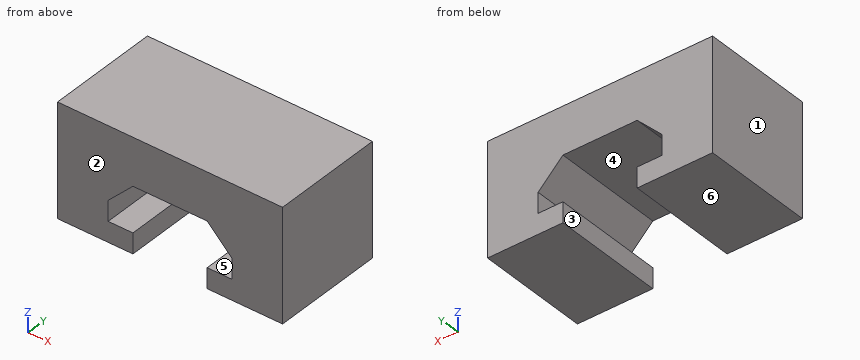
```python
from build123d import *

# Parameters (mm, degrees)
SKETCH_W     = 20
SKETCH_H     = 10
PAD_DEPTH    = 10
POCKET_DEPTH = 10.001


with BuildPart() as part:
    # Sketch → Pad (new body)
    with BuildSketch(Plane.XZ):
        with Locations((0, 5)):
            Rectangle(SKETCH_W, SKETCH_H)
    extrude(amount=PAD_DEPTH)

    # Sketch001 (on Face6 of Pad) → Pocket (cut, through all)
    with BuildSketch(Plane.XZ.offset(10)):
        Polygon((-3.3, 0), (3.3, 0), (3.3, 1.8), (5.5, 1.8), (5.5, 3.6), (3.3, 5.8), (-3.3, 5.8), (-5.5, 3.6), (-5.5, 1.8), (-3.3, 1.8), align=None)
    extrude(amount=-POCKET_DEPTH, mode=Mode.SUBTRACT)


solid = part.part
```
The model under review builds one solid part; all positions refer to its coordinate system, in mm. Face numbers are marked on the shaded views. A direction names the side the tool comes from. Coordinates: 2 decimals unless noted, no trailing zeros. Order: outer loops, then holes, each group sorted by start corner. A loop starts at its lowest first (then second) coordinate and runs counter-clockwise, first axis right, second up. Notation, with made-up numbers: (23, 70) -> (38, 70) arc R23 cw to (38, 90) -> close; hole circle Ø7 at (46, -13.5). An arc over 180 degrees is marked (long way). Answer in a Markdown table with one row per item. Add a question column.
Item 1: Machinability: for the marked faces 4, 5 and 6, which of the approach directions +Z, -Z, +X, -X, +Y, -Y give a long, thin tool a straight path to every point of the face, cutting with its end or side? Answer none if there is none.
Item 2: We need section A-A on x = -3.5. Write out the cut boundary in (y, z), plus the area to 3 significant figures.
Item 3: We need section B-B on z = 3. Write out the cut boundary in (x, y), plus the area to 3 significant figures.
Item 4: We need section C-C on y = -8. Write out the cut boundary in (x, z).
Item 5: Mouldability with a two-part tool opening along X and no side actions: class the marked faces 1, 2 and 3 as +X half, -X half, draft (parallel to the pull), parting line (faces both ways), or undercut.
Item 6: To check wall thickness, follow probe 1 along X at (y, z) = (-0.5, 2); probe 2 along X at (y, z) = (-5, 0.5); probe 3 along Z at (x, y) = (-0.25, -8.5). State the ranges of each line that lie inside material, in increasing order.
Final values:
| question | item | result |
|---|---|---|
| 1 | face 4 | -Z, +Y, -Y |
| 1 | face 5 | +Y, -Y |
| 1 | face 6 | -Z, +X, -X, +Y, -Y |
| 2 | outline | (-10, 0) -> (0, 0) -> (0, 1.8) -> (-10, 1.8) -> close; (-10, 5.6) -> (0, 5.6) -> (0, 10) -> (-10, 10) -> close |
| 2 | area | 62.0 mm2 |
| 3 | outline | (-10, -10) -> (-5.5, -10) -> (-5.5, 0) -> (-10, 0) -> close; (5.5, -10) -> (10, -10) -> (10, 0) -> (5.5, 0) -> close |
| 3 | area | 90.0 mm2 |
| 4 | outline | (-10, 0) -> (-3.3, 0) -> (-3.3, 1.8) -> (-5.5, 1.8) -> (-5.5, 3.6) -> (-3.3, 5.8) -> (3.3, 5.8) -> (5.5, 3.6) -> (5.5, 1.8) -> (3.3, 1.8) -> (3.3, 0) -> (10, 0) -> (10, 10) -> (-10, 10) -> close |
| 5 | face 1 | -X half |
| 5 | face 2 | draft |
| 5 | face 3 | undercut |
| 6 | probe 1 | x = -10 to -5.5, 5.5 to 10 |
| 6 | probe 2 | x = -10 to -3.3, 3.3 to 10 |
| 6 | probe 3 | z = 5.8 to 10 |
